Verification items for the finished model (mm, model axes). Round coordinates to 2 decimals unless told otherwise and drop trailing zeros. Loops run counter-clockwise (first coordinate to the right, second up) from the corner with the lowest first, then second, coordinate; pieces in that order, holes last. Notation, with made-up numbers: (-39, 72.5) - (13, 72.5) arc R10 ccw to (13, 89.5) - close; hole circle Ø2 at (-22.75, 63). An arc over 180 degrees is marked (long way). Use a Markdown table: item, result. Add a question column.
```python
from build123d import *

# Parameters (mm, degrees)
SZKIC1_W                    = 25
SZKIC1_H                    = 15
SZKIC1_R                    = 1.65
DODANIE_WYCI_GNI_CIE1_DEPTH = 5
SZKIC2_R                    = 1.55
WYTNIJ_WYCI_GNI_CIE1_DEPTH  = 5


with BuildPart() as part:
    # Szkic1 → Dodanie-wyciągnięcie1 (new body)
    with BuildSketch(Plane.XY):
        with Locations((8.5, 3.5)):
            Rectangle(SZKIC1_W, SZKIC1_H)
        Circle(SZKIC1_R, mode=Mode.SUBTRACT)
        with Locations((0, 7)):
            Circle(SZKIC1_R, mode=Mode.SUBTRACT)
        with Locations((17, 0)):
            Circle(SZKIC1_R, mode=Mode.SUBTRACT)
        with Locations((17, 7)):
            Circle(SZKIC1_R, mode=Mode.SUBTRACT)
    extrude(amount=DODANIE_WYCI_GNI_CIE1_DEPTH)

    # Szkic2 → Wytnij-wyciągnięcie1 (cut)
    with BuildSketch(Plane.XY.offset(5)):
        with Locations((8.5, 5.5)):
            Circle(SZKIC2_R)
    extrude(amount=-WYTNIJ_WYCI_GNI_CIE1_DEPTH, mode=Mode.SUBTRACT)


solid = part.part
```
Q1. Thickness scan on line 1 along Y through (x, z) = (0, 3.65); line 2 along X through (y, z) = (8.5, 0.6); line 3 along Y through (x, z) = (8.5, 3). Record the ranges inside material, lowest first.
Q2. Section check C-C on x = 8.5. Record the cut outline in (y, z).
Q3. Release check for a two-part mould opening along Y. For faces 1 (the face through (-4, 3, 2)), 2 (the face through (8, 11, 2)), 3 (the face through (-0.4, 5.4, 2.5)) record: +Y half, -Y half, draft (parallel to the pull), parting line (faces both ways), or undercut.
Q4. Section check D-D on z = 2.2. Record the cut outline in (x, y).
Q5. Section check B-B on y = 0. Record the cut outline in (x, z).
Q6. Section check A-A on x = 0. Record the cut outline in (y, z).
Determined:
| question | item | result |
|---|---|---|
| 1 | line 1 | y = -4 to -1.65, 1.65 to 5.35, 8.65 to 11 |
| 1 | line 2 | x = -4 to -0.69, 0.69 to 16.31, 17.69 to 21 |
| 1 | line 3 | y = -4 to 3.95, 7.05 to 11 |
| 2 | outline | (-4, 0) - (3.95, 0) - (3.95, 5) - (-4, 5) - close; (7.05, 0) - (11, 0) - (11, 5) - (7.05, 5) - close |
| 3 | face 1 | draft |
| 3 | face 2 | +Y half |
| 3 | face 3 | undercut |
| 4 | outline | (-4, -4) - (21, -4) - (21, 11) - (-4, 11) - close; hole circle Ø3.3 at (0, 0); hole circle Ø3.3 at (0, 7); hole circle Ø3.1 at (8.5, 5.5); hole circle Ø3.3 at (17, 0); hole circle Ø3.3 at (17, 7) |
| 5 | outline | (-4, 0) - (-1.65, 0) - (-1.65, 5) - (-4, 5) - close; (1.65, 0) - (15.35, 0) - (15.35, 5) - (1.65, 5) - close; (18.65, 0) - (21, 0) - (21, 5) - (18.65, 5) - close |
| 6 | outline | (-4, 0) - (-1.65, 0) - (-1.65, 5) - (-4, 5) - close; (1.65, 0) - (5.35, 0) - (5.35, 5) - (1.65, 5) - close; (8.65, 0) - (11, 0) - (11, 5) - (8.65, 5) - close |
